Can you work these out from the model? Positions are in its coordinate system, mm. A direction names the side the tool comes from. Give positions to 0.01 mm unless a question says otherwise; leave off trailing zeros. Order: outer loops, then holes, each group sorted by start corner. A loop starts at its lowest first (then second) coordinate and runs counter-clockwise, first axis right, second up. Notation, with made-up numbers: (80, 54) - (114, 54) arc R25 ccw to (114, 81) - close; hole circle Ø6 at (-22, 19.25). An arc over 180 degrees is marked (long way). One line per question, with ' | ' between items.
```python
from build123d import *

# Parameters (mm, degrees)
SKETCH1_W           = 20
SKETCH1_H           = 20
BOSS_EXTRUDE1_DEPTH = 30
FILLET1_R           = 2
SKETCH2_R           = 1
CUT_EXTRUDE1_DEPTH  = 3
SKETCH3_R           = 7.5
BOSS_EXTRUDE2_DEPTH = 1.5
SKETCH4_R           = 2.38
BOSS_EXTRUDE3_DEPTH = 100


with BuildPart() as part:
    # Sketch1 → Boss-Extrude1 (new body)
    with BuildSketch(Plane(origin=(0, 0, 0), x_dir=(1, 0, 0), z_dir=(0, 1, 0))):
        Rectangle(SKETCH1_W, SKETCH1_H)
    extrude(amount=BOSS_EXTRUDE1_DEPTH)

    # Fillet1
    fillet1_edges = [part.edges().sort_by_distance(p)[0] for p in [
        (10, 15, 10),
        (-10, 15, 10),
        (-10, 15, -10),
        (10, 15, -10),
    ]]
    fillet(fillet1_edges, radius=FILLET1_R)

    # Sketch2 → Cut-Extrude1 (cut)
    with BuildSketch(Plane(origin=(0, 30, 0), x_dir=(1, 0, 0), z_dir=(0, 1, 0))):
        with Locations(Location((-8, 8, 0), (0, 0, 270))):
            Circle(SKETCH2_R)
        with Locations(Location((8, 8, 0), (0, 0, 270))):
            Circle(SKETCH2_R)
        with Locations(Location((8, -8, 0), (0, 0, 270))):
            Circle(SKETCH2_R)
        with Locations(Location((-8, -8, 0), (0, 0, 270))):
            Circle(SKETCH2_R)
    extrude(amount=-CUT_EXTRUDE1_DEPTH, mode=Mode.SUBTRACT)

    # Sketch3 → Boss-Extrude2 (add)
    with BuildSketch(Plane(origin=(0, 30, 0), x_dir=(1, 0, 0), z_dir=(0, 1, 0))):
        with Locations(Location((0, 0, 0), (0, 0, 90))):
            Circle(SKETCH3_R)
    extrude(amount=BOSS_EXTRUDE2_DEPTH)

    # Sketch4 → Boss-Extrude3 (add)
    with BuildSketch(Plane(origin=(0, 31.5, 0), x_dir=(1, 0, 0), z_dir=(0, 1, 0))):
        with Locations(Location((0, 0, 0), (0, 0, 270))):
            Circle(SKETCH4_R)
    extrude(amount=BOSS_EXTRUDE3_DEPTH)


solid = part.part
```
(1) Imagine slicing it at A-A (z = 0). List the corners of the cut face in (x, y) for me, and give its area (3 significant figures).
Answer below:
outline: (-10, 0) - (10, 0) - (10, 30) - (7.5, 30) - (7.5, 31.5) - (2.38, 31.5) - (2.38, 131.5) - (-2.38, 131.5) - (-2.38, 31.5) - (-7.5, 31.5) - (-7.5, 30) - (-10, 30) - close | area: 1,100 mm^2
(2) On a 3-axis mill with a long thin cutter (end or side, diameter ignored), from which of +Z, -Z, +X, -X, +Y, -Y can I reach the whole of each face in a straight line? I mean faces 1 (the face through (-0.33, 30.74, 7.493)), 2 (the face through (0, 0, 0)). Say none if no direction works.
Answer below:
face 1: +Y | face 2: +Z, -Z, +X, -X, -Y
(3) Imagine slicing it at D-D (z = 5.5). List the corners of the cut face in (x, y) for me.
Answer below:
outline: (-10, 0) - (10, 0) - (10, 30) - (5.1, 30) - (5.1, 31.5) - (-5.1, 31.5) - (-5.1, 30) - (-10, 30) - close
(4) Imagine slicing it at B-B (x = 0). List the corners of the cut face in (y, z) for me, and give its area (3 significant figures).
Answer below:
outline: (0, -10) - (30, -10) - (30, -7.5) - (31.5, -7.5) - (31.5, -2.38) - (131.5, -2.38) - (131.5, 2.38) - (31.5, 2.38) - (31.5, 7.5) - (30, 7.5) - (30, 10) - (0, 10) - close | area: 1,100 mm^2
(5) Imagine slicing it at C-C (y = 124.5). List the corners of the cut face in (x, z) for me, and give its area (3 significant figures).
Answer below:
outline: circle Ø4.76 at (0, 0) | area: 17.8 mm^2
(6) Will these pins go through, and if not, where does the flat tip stop? pin 1 (1 mm diameter, centred on x = 0, z = 4, fed in from +Y); pin 2 (2 mm diameter, centred on x = 8, z = -7.5, fed in from +Y); pin 3 (10 mm diameter, centred on x = -6, y = 109.5, fed in from +Z).
Answer below:
pin 1: y = 31.5 | pin 2: y = 30 | pin 3: z = 2.16
(7) If I drill on line 1 (X direction, y = 27.7, z = 8); line 2 (Y direction, x = 7.25, z = -5.75); line 3 (Y direction, x = 4, z = -5.25), over which ranges is the centre line in solid material (lowest first)?
Answer below:
line 1: -10 to -9, -7 to 7, 9 to 10 | line 2: 0 to 30 | line 3: 0 to 31.5
